from build123d import *

# Parameters (mm, degrees)
F0_R          = 3
F0_R_2        = 2.5
F1_DEPTH      = 251
F2_R          = 2
F3_R          = 7
F6_DEPTH      = 30
F6_DEPTH_BACK = 30


# Not quite as in the source:
# - a feature names something its author has since deleted; it is built from what else it names


with BuildPart() as f1:
    # F0 (on Top) → F1 (new body)
    with BuildSketch(Plane.XY):
        with BuildLine():
            Line((18.15, -30), (30, -30))
            Line((30, -30), (30, -18.15))
            Line((30, -18.15), (27.5, -18.15))
            Line((27.5, -18.15), (27.5, -20.15))
            Line((27.5, -20.15), (21.5477069044, -20.15))
            ThreePointArc((21.5477069044, -20.15), (19.5, -15), (21.5477069044, -9.85))
            Line((21.5477069044, -9.85), (27.5, -9.85))
            Line((27.5, -9.85), (27.5, -11.85))
            Line((27.5, -11.85), (30, -11.85))
            Line((30, -11.85), (30, 11.85))
            Line((30, 11.85), (27.5, 11.85))
            Line((27.5, 11.85), (27.5, 9.85))
            Line((27.5, 9.85), (21.5477069044, 9.85))
            ThreePointArc((21.5477069044, 9.85), (19.5, 15), (21.5477069044, 20.15))
            Line((21.5477069044, 20.15), (27.5, 20.15))
            Line((27.5, 20.15), (27.5, 18.15))
            Line((27.5, 18.15), (30, 18.15))
            Line((30, 18.15), (30, 30))
            Line((30, 30), (18.15, 30))
            Line((18.15, 30), (18.15, 27.5))
            Line((18.15, 27.5), (20.15, 27.5))
            Line((20.15, 27.5), (20.15, 21.5477069044))
            ThreePointArc((20.15, 21.5477069044), (15, 19.5), (9.85, 21.5477069044))
            Line((9.85, 21.5477069044), (9.85, 27.5))
            Line((9.85, 27.5), (11.85, 27.5))
            Line((11.85, 27.5), (11.85, 30))
            Line((11.85, 30), (-11.85, 30))
            Line((-11.85, 30), (-11.85, 27.5))
            Line((-11.85, 27.5), (-9.85, 27.5))
            Line((-9.85, 27.5), (-9.85, 21.5477069044))
            ThreePointArc((-9.85, 21.5477069044), (-15, 19.5), (-20.15, 21.5477069044))
            Line((-20.15, 21.5477069044), (-20.15, 27.5))
            Line((-20.15, 27.5), (-18.15, 27.5))
            Line((-18.15, 27.5), (-18.15, 30))
            Line((-18.15, 30), (-30, 30))
            Line((-30, 30), (-30, 18.15))
            Line((-30, 18.15), (-27.5, 18.15))
            Line((-27.5, 18.15), (-27.5, 20.15))
            Line((-27.5, 20.15), (-21.5477069044, 20.15))
            ThreePointArc((-21.5477069044, 20.15), (-19.5, 15), (-21.5477069044, 9.85))
            Line((-21.5477069044, 9.85), (-27.5, 9.85))
            Line((-27.5, 9.85), (-27.5, 11.85))
            Line((-27.5, 11.85), (-30, 11.85))
            Line((-30, 11.85), (-30, -11.85))
            Line((-30, -11.85), (-27.5, -11.85))
            Line((-27.5, -11.85), (-27.5, -9.85))
            Line((-27.5, -9.85), (-21.5477069044, -9.85))
            ThreePointArc((-21.5477069044, -9.85), (-19.5, -15), (-21.5477069044, -20.15))
            Line((-21.5477069044, -20.15), (-27.5, -20.15))
            Line((-27.5, -20.15), (-27.5, -18.15))
            Line((-27.5, -18.15), (-30, -18.15))
            Line((-30, -18.15), (-30, -30))
            Line((-30, -30), (-18.15, -30))
            Line((-18.15, -30), (-18.15, -27.5))
            Line((-18.15, -27.5), (-20.15, -27.5))
            Line((-20.15, -27.5), (-20.15, -21.5477069044))
            ThreePointArc((-20.15, -21.5477069044), (-15, -19.5), (-9.85, -21.5477069044))
            Line((-9.85, -21.5477069044), (-9.85, -27.5))
            Line((-9.85, -27.5), (-11.85, -27.5))
            Line((-11.85, -27.5), (-11.85, -30))
            Line((-11.85, -30), (11.85, -30))
            Line((11.85, -30), (11.85, -27.5))
            Line((11.85, -27.5), (9.85, -27.5))
            Line((9.85, -27.5), (9.85, -21.5477069044))
            ThreePointArc((9.85, -21.5477069044), (15, -19.5), (20.15, -21.5477069044))
            Line((20.15, -21.5477069044), (20.15, -27.5))
            Line((20.15, -27.5), (18.15, -27.5))
            Line((18.15, -27.5), (18.15, -30))
        make_face()
        with Locations((-25, -25)):
            Circle(F0_R, mode=Mode.SUBTRACT)
        with Locations((-15, -15)):
            Circle(F0_R_2, mode=Mode.SUBTRACT)
        with Locations((25, -25)):
            Circle(F0_R, mode=Mode.SUBTRACT)
        with Locations((15, -15)):
            Circle(F0_R_2, mode=Mode.SUBTRACT)
        with Locations((-25, 25)):
            Circle(F0_R, mode=Mode.SUBTRACT)
        with Locations((-15, 15)):
            Circle(F0_R_2, mode=Mode.SUBTRACT)
        Polygon((-7, 22), (-7, 27.5), (0, 27.5), (7, 27.5), (7, 22), (10, 16), (10, 10), (16, 10), (22, 7), (27.5, 7), (27.5, 0), (27.5, -7), (22, -7), (16, -10), (10, -10), (10, -16), (7, -22), (7, -27.5), (0, -27.5), (-7, -27.5), (-7, -22), (-10, -16), (-10, -10), (-16, -10), (-22, -7), (-27.5, -7), (-27.5, 0), (-27.5, 7), (-22, 7), (-16, 10), (-10, 10), (-10, 16), align=None, mode=Mode.SUBTRACT)
        with Locations((15, 15)):
            Circle(F0_R_2, mode=Mode.SUBTRACT)
        with Locations((25, 25)):
            Circle(F0_R, mode=Mode.SUBTRACT)
    extrude(amount=F1_DEPTH)

    # F2
    f2_edges = [f1.edges().sort_by_distance(p)[0] for p in [
        (-7, 27.5, 125.5),
        (7, 27.5, 125.5),
    ]]
    fillet(f2_edges, radius=F2_R)

    # F3
    f3_edges = [f1.edges().sort_by_distance(p)[0] for p in [
        (-10, 16, 125.5),
        (10, 16, 125.5),
    ]]
    fillet(f3_edges, radius=F3_R)

    # F5 (on Front) → F6 (cut, two sides)
    with BuildSketch(Plane.XZ) as f6_sk:
        Polygon((-177.8936772938, 164.8876193333), (30, 251), (-52.9032198334, 451.1460776863), (-260.7968971272, 365.0336970195), align=None)
        Polygon((247.13668536, 46.6947819077), (131.9157336339, 161.9157336339), (-30, 0), (85.2209517261, -115.2209517261), align=None)
    extrude(amount=F6_DEPTH, mode=Mode.SUBTRACT)
    extrude(f6_sk.sketch, amount=-F6_DEPTH_BACK, mode=Mode.SUBTRACT)


solid = f1.part
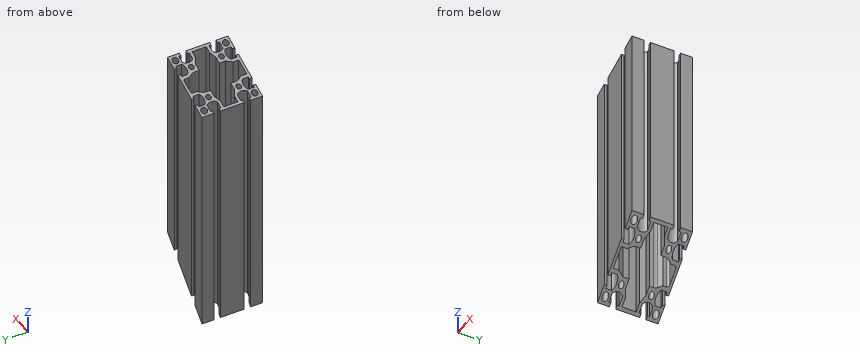
Read the model definition and answer for the solid it produces. Units are mm, in the model's axes. Round coordinates to 2 decimals unless told otherwise and drop trailing zeros. Write each loop counter-clockwise with the first axis right and the second up, starting at its lowest first coordinate (ties: lowest second). Pieces come first, ordered by that corner, then holes. Notation, with made-up numbers: (83.25, 47) - (125.25, 47) arc R29 cw to (125.25, 68) - close; hole circle Ø2 at (31, -8). An arc over 180 degrees is marked (long way). One line per question, with ' | ' between items. Start each with the question number.
1. Each of these flat-tipped pins is pushed along its axis until it touches: pin 1 (8 mm diameter, centred on x = -15, y = -15, fed in from -Z); pin 2 (2 mm diameter, centred on y = 17.5, z = 53.5, fed in from +X); pin 3 (4 mm diameter, centred on x = -12.5, y = -12.5, fed in from +Z). Where does it stop, or does it pass through?
2. Section C-C (x = 0.5) is taken. Determine the outline of the cut face in (y, z), and give its area (3 significant figures).
3. Section A-A (x = -25) is taken. Determine the outline of the cut face in (y, z).
4. Find the intervals of material crossed by probe 1 along Y at (x, z) = (25, 144); probe 2 along Y at (x, z) = (-15, 136), in increasing order. Write a range as [from, to].
5. Section B-B (z = 55) is taken. Give the number of separate pieces and of enclosed holes in the cut face, and give its area (3 significant figures).
Filled in:
1) pin 1: z = 11 | pin 2: x = 20.37 | pin 3: z = 234.22
2) outline: (-30, 30.5) - (-27.5, 30.5) - (-27.5, 238.78) - (-30, 238.78) - close; (27.5, 30.5) - (30, 30.5) - (30, 238.78) - (27.5, 238.78) - close | area: 1,040 mm²
3) outline: (-30, 5) - (-28, 5) - (-28, 228.22) - (-30, 228.22) - close; (-22, 5) - (-20.15, 5) - (-20.15, 228.22) - (-22, 228.22) - close; (-9.85, 5) - (-7, 5) - (-7, 228.22) - (-9.85, 228.22) - close; (7, 5) - (9.85, 5) - (9.85, 228.22) - (7, 228.22) - close; (20.15, 5) - (22, 5) - (22, 228.22) - (20.15, 228.22) - close; (28, 5) - (30, 5) - (30, 228.22) - (28, 228.22) - close
4) probe 1: [-30, -28], [-22, -20.15], [-9.85, -7], [7, 9.85], [20.15, 22], [28, 30] | probe 2: [-19.5, -17.5], [-12.5, -10], [10, 12.5], [17.5, 19.5]
5) separate pieces: 1 | enclosed holes: 6 | area: 928 mm²
